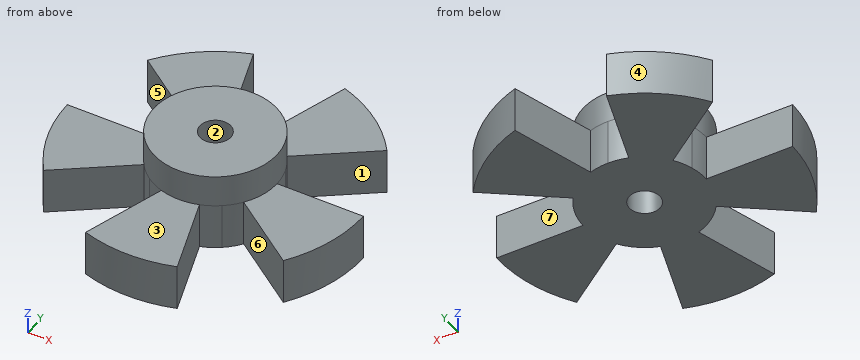
```python
from build123d import *
from build123d.topology import SkipClean

# Parameters (mm, degrees)
SZKIC1_R                    = 4.8
DODANIE_WYCI_GNI_CIE1_DEPTH = 1.5
SZKIC2_R                    = 2
DODANIE_WYCI_GNI_CIE2_DEPTH = 1.5
WYTNIJ_WYCI_GNI_CIE1_REACH  = 8.952
SZYK_KO_OWY2_COUNT          = 5
OTW_R1_D                    = 1
ESBO_O1_R                   = 2
CORTE_EXTRUS_O1_DEPTH       = 0.46


with BuildPart() as part:
    # Szkic1 → Dodanie-wyci_gni_cie1 (new body)
    with BuildSketch(Plane.XY):
        Circle(SZKIC1_R)
    extrude(amount=DODANIE_WYCI_GNI_CIE1_DEPTH)

    # Szkic2 → Dodanie-wyci_gni_cie2 (add)
    with BuildSketch(Plane.XY.offset(1.5)):
        Circle(SZKIC2_R)
    extrude(amount=DODANIE_WYCI_GNI_CIE2_DEPTH)

    # Szkic3 → Wytnij-wyci_gni_cie1 (cut, up to next)
    with BuildSketch(Plane.XY.offset(1.5), mode=Mode.PRIVATE) as wytnij_wyci_gni_cie1_sk1:
        with BuildLine():
            ThreePointArc((-0.618033989, 1.902113033), (-0.31286893, 1.975376681), (0, 2))
            Line((0, 2), (0, 4.8))
            ThreePointArc((0, 4.8), (-0.750885432, 4.740904035), (-1.483281573, 4.565071278))
            Line((-1.483281573, 4.565071278), (-0.618033989, 1.902113033))
        make_face()
    wytnij_wyci_gni_cie1_tool1 = extrude(wytnij_wyci_gni_cie1_sk1.sketch, amount=-WYTNIJ_WYCI_GNI_CIE1_REACH, mode=Mode.PRIVATE) & part.part
    # Szkic3 → Wytnij-wyci_gni_cie1 (cut, up to next)
    with BuildSketch(Plane.XY.offset(1.5), mode=Mode.PRIVATE) as wytnij_wyci_gni_cie1_sk2:
        with BuildLine():
            Line((0, 4.8), (0, 2))
            ThreePointArc((0, 2), (0.31286893, 1.975376681), (0.618033989, 1.902113033))
            Line((0.618033989, 1.902113033), (1.483281573, 4.565071278))
            ThreePointArc((1.483281573, 4.565071278), (0.750885432, 4.740904035), (0, 4.8))
        make_face()
    wytnij_wyci_gni_cie1_tool2 = extrude(wytnij_wyci_gni_cie1_sk2.sketch, amount=-WYTNIJ_WYCI_GNI_CIE1_REACH, mode=Mode.PRIVATE) & part.part
    wytnij_wyci_gni_cie1_1 = wytnij_wyci_gni_cie1_tool1.solids().sort_by_distance((-0.559629, 3.533359, 1.5))[0]
    add(wytnij_wyci_gni_cie1_1, mode=Mode.SUBTRACT)
    wytnij_wyci_gni_cie1_2 = wytnij_wyci_gni_cie1_tool2.solids().sort_by_distance((0.559629, 3.533359, 1.5))[0]
    add(wytnij_wyci_gni_cie1_2, mode=Mode.SUBTRACT)
    wytnij_wyci_gni_cie1 = wytnij_wyci_gni_cie1_1 + wytnij_wyci_gni_cie1_2  # Wytnij-wyci_gni_cie1 as one shape, for the pattern or mirror that repeats it

    # Szyk ko_owy2: Wytnij-wyci_gni_cie1 ×5 about axis
    with SkipClean():  # the faces are left unmerged after this step: merging them gives an invalid solid
        szyk_ko_owy2_axis = Axis((0, 0, 0), (0, 0, 1))
        for i in range(1, SZYK_KO_OWY2_COUNT):
            add(wytnij_wyci_gni_cie1.rotate(szyk_ko_owy2_axis, i * 360 / SZYK_KO_OWY2_COUNT), mode=Mode.SUBTRACT)

    # Otw_r1 (through all)
    with Locations(Plane.XY.offset(3)):
        with Locations((0, 0)):
            Hole(OTW_R1_D / 2)

    # Esbo_o1 → Corte-extrus_o1 (cut)
    with SkipClean():  # the faces are left unmerged after this step: merging them gives an invalid solid
        with BuildSketch(Plane.XY.offset(3)):
            Circle(ESBO_O1_R)
        extrude(amount=-CORTE_EXTRUS_O1_DEPTH, mode=Mode.SUBTRACT)


solid = part.part
```
The listing builds one solid part. Answer for the finished solid, in the listing's coordinates (mm). Face numbers are marked on the shaded views. A direction names the side the tool comes from. Coordinates: 2 decimals unless noted, no trailing zeros. Write each loop counter-clockwise with the first axis right and the second up, starting at its lowest first coordinate (ties: lowest second). Pieces come first, ordered by that corner, then holes. Notation, with made-up numbers: (-13, 83) - (-6, 83) arc R27 ccw to (-6, 104) - close; hole circle Ø4 at (-39.75, 21.25). An arc over 180 degrees is marked (long way). Return JSON: item names as keys, results as strings. Group by question number.
Q1. The part is cut by section C-C on y = 3.75. Write down the section's boundary in (x, z), and give its area (3 significant figures).
Q2. For a pull along X with two mould halves and no side action, classify the marked faces 1, 2, 3 and 4 as +X half, -X half, draft (parallel to the pull), parting line (faces both ways), or undercut.
Q3. Flat-ended cylindrical pins translate along their axes: pin 1 Ø0.8 at (x, z) = (-3, 1) entering from +Y; pin 2 Ø3 at (x, y) = (0, -4) entering from +Z; pin 3 Ø0.8 at (x, z) = (3.5, 0.5) entering from +Y. Find the tip coordinate at first contact, or state that the pin passes through.
Q4. The part is cut by section A-A on z = 0.2. Write down the section's boundary in (x, y), and give its area (3 significant figures).
Q5. Which of the six approach directions +Z, -Z, +X, -X, +Y, -Y give full straight-line access (tool end or side, diameter ignored) to the marked faces 5, 6 and 7?
Q6. The part is cut by section B-B on x = 3.5. Write down the section's boundary in (y, z), and give its area (3 significant figures).
Q7. The part is cut by section D-D on x = -0.75. Write down the section's boundary in (y, z).
Q8. Find the intervals of material crossed by line 1 along Y through (x, z) = (0, 0.6); line 2 along Z through (x, y) = (-3, -0.25); line 3 along X through (y, z) = (3.75, 0.7), in increasing order. Write a range as [from, to].
Evaluation:
{
 "1": {"outline": "(-3, 0) - (-1.22, 0) - (-1.22, 1.5) - (-3, 1.5) - close; (1.22, 0) - (3, 0) - (3, 1.5) - (1.22, 1.5) - close", "area": "5.33 mm2"},
 "2": {"face 1": "+X half", "face 2": "undercut", "face 3": "draft", "face 4": "-X half"},
 "3": {"pin 1": "stops at y = 4.03", "pin 2": "stops at z = 1.5", "pin 3": "stops at y = 3.66"},
 "4": {"outline": "(-4.8, 0) arc R4.8 ccw to (-3.88, -2.82) - (-1.62, -1.18) arc R2 ccw to (-0.62, -1.9) - (-1.48, -4.57) arc R4.8 ccw to (1.48, -4.57) - (0.62, -1.9) arc R2 ccw to (1.62, -1.18) - (3.88, -2.82) arc R4.8 ccw to (4.8, 0) - (2, 0) arc R2 ccw to (1.62, 1.18) - (3.88, 2.82) arc R4.8 ccw to (1.48, 4.57) - (0.62, 1.9) arc R2 ccw to (-0.62, 1.9) - (-1.48, 4.57) arc R4.8 ccw to (-3.88, 2.82) - (-1.62, 1.18) arc R2 ccw to (-2, 0) - close; hole circle Ø1 at (0, 0)", "area": "41.7 mm2"},
 "5": {"face 5": "+Z, -Z, -X", "face 6": "+Z, -Z, -Y", "face 7": "+Z, -Z, +X"},
 "6": {"outline": "(-2.54, 0) - (0, 0) - (0, 1.5) - (-2.54, 1.5) - close; (2.54, 0) - (3.28, 0) - (3.28, 1.5) - (2.54, 1.5) - close", "area": "4.93 mm2"},
 "7": {"outline": "(-4.74, 0) - (-2.31, 0) - (-2.31, 1.5) - (-4.74, 1.5) - close; (-1.85, 0) - (2.31, 0) - (2.31, 1.5) - (1.85, 1.5) - (1.85, 2.54) - (-1.85, 2.54) - close"},
 "8": {"line 1": "y = [-4.8, -0.5], [0.5, 2]", "line 2": "z = [0, 1.5]", "line 3": "x = [-3, -1.22], [1.22, 3]"}
}
